Check sheet for the modelled part. Datum: model origin and axes. Units: mm. Face numbers are marked on the shaded views. Give positions to 0.01 mm unless a question says otherwise; leave off trailing zeros. Loops run counter-clockwise (first coordinate to the right, second up) from the corner with the lowest first, then second, coordinate; pieces in that order, holes last. Notation, with made-up numbers: (-9.75, -23) - (35.25, -23) arc R13 cw to (35.25, -13) - close; hole circle Ø5 at (37, -28). An arc over 180 degrees is marked (long way). Answer in a Markdown table with one row per item. Add a question column.
(1) Go/stop test with a flat-tipped pin: P1, Ø1.5, axis at y = 0, z = 0, coming from the +X side. Record where the tip stops, or that it passes through.
(2) Sectioned sample at B-B on x = -4. Enter the section's corners in (y, z).
(3) Sectioned sample at A-A on x = 3.75. Enter the section's corners in (y, z).
(4) Thickness scan on L1, parallel to Y at x = -1, z = 0; L2, parallel to Y at x = -1.25, z = 0.55. Record the ranges inside material, lowest first.
(5) Draft check along Y on the marked faces 1, 2 and 3. Enter one of: released by +Y, released by -Y, zero draft, split by the parting line, or undercut.
from build123d import *

# Parameters (mm, degrees)
SKETCH1_R                 = 2.75
BOSS_EXTRUDE1_DEPTH       = 5
CHAMFER1_SIZE             = 0.2
M3X0_5_TAPPED_HOLE1_D     = 2.5
M3X0_5_TAPPED_HOLE1_DEPTH = 7.5
M3X0_5_TAPPED_HOLE1_TIP   = 0.751075774


with BuildPart() as part:
    # Sketch1 → Boss-Extrude1 (new body, symmetric)
    with BuildSketch(Plane(origin=(0, 0, 0), x_dir=(0, -1, 0), z_dir=(1, 0, 0))):
        Circle(SKETCH1_R)
    extrude(amount=BOSS_EXTRUDE1_DEPTH, both=True)

    # Chamfer1
    chamfer1_edges = [part.edges().sort_by_distance(p)[0] for p in [
        (-5, 2.75, 0),
        (5, 2.75, 0),
    ]]
    chamfer(chamfer1_edges, length=CHAMFER1_SIZE)

    # M3x0.5 Tapped Hole1
    with Locations(Plane(origin=(5, 0, 0), x_dir=(0, 0, -1), z_dir=(1, 0, 0))):
        with Locations((0, 0)):
            Hole(M3X0_5_TAPPED_HOLE1_D / 2, depth=M3X0_5_TAPPED_HOLE1_DEPTH)
            with Locations((0, 0, -(M3X0_5_TAPPED_HOLE1_DEPTH + M3X0_5_TAPPED_HOLE1_TIP / 2))):  # 118° drill point
                Cone(0, M3X0_5_TAPPED_HOLE1_D / 2, M3X0_5_TAPPED_HOLE1_TIP, mode=Mode.SUBTRACT)


solid = part.part
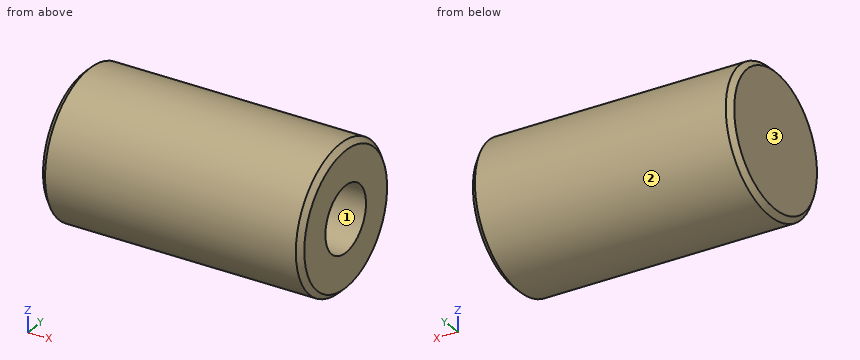
Reply:
| question | item | result |
|---|---|---|
| 1 | P1 | x = -2.8 |
| 2 | outline | circle Ø5.5 at (0, 0) |
| 3 | outline | circle Ø5.5 at (0, 0); hole circle Ø2.5 at (0, 0) |
| 4 | L1 | -2.75 to -1.25, 1.25 to 2.75 |
| 4 | L2 | -2.69 to -1.12, 1.12 to 2.69 |
| 5 | face 1 | undercut |
| 5 | face 2 | split by the parting line |
| 5 | face 3 | zero draft |
